from build123d import *

# Parameters (mm, degrees)
F0_R     = 1.8415
F1_DEPTH = 12.7


with BuildPart() as f1:
    # F0 (on Top) → F1 (new body, symmetric)
    with BuildSketch(Plane.XY):
        with BuildLine():
            Line((9.525, 12.7), (-9.525, 12.7))
            ThreePointArc((-9.525, 12.7), (-11.770064, 11.770064), (-12.7, 9.525))
            Line((-12.7, 9.525), (-12.7, -9.525))
            ThreePointArc((-12.7, -9.525), (-11.770064, -11.770064), (-9.525, -12.7))
            Line((-9.525, -12.7), (9.525, -12.7))
            ThreePointArc((9.525, -12.7), (11.770064, -11.770064), (12.7, -9.525))
            Line((12.7, -9.525), (12.7, 9.525))
            ThreePointArc((12.7, 9.525), (11.770064, 11.770064), (9.525, 12.7))
        make_face()
        Circle(F0_R, mode=Mode.SUBTRACT)
    extrude(amount=F1_DEPTH, both=True)


solid = f1.part
Source: CAD feature listing. Evaluate the final solid. Frame: model axes, mm. Round coordinates to 2 decimals unless told otherwise and drop trailing zeros. Loops run counter-clockwise (first coordinate to the right, second up) from the corner with the lowest first, then second, coordinate; pieces in that order, holes last.
Q1. Mould query, pull axis X, two halves, no side actions, for faces 1 (the face through (-11.79, -11.75, 0.18)), 2 (the face through (0, -12.7, 0)), 3 (the face through (0.85, -1.634, -0.178)). Classes: pulls with the +X half, pulls with the -X half, needs draft (parallel to the pull), parting line crosses it, or undercut.
Q2. Ray query, line 1 (Y direction, x = 0, z = -6.75); line 2 (Y direction, x = -9.75, z = -2.5); line 3 (X direction, y = -0.25, z = 5.75). Return the intervals inside material, ascending.
Q3. Section A-A, the plane y = 0. Return loops of the section in (x, z).
Solutions:
1. face 1: pulls with the -X half
1. face 2: needs draft
1. face 3: undercut
2. line 1: y = -12.7 to -1.84, 1.84 to 12.7
2. line 2: y = -12.69 to 12.69
2. line 3: x = -12.7 to -1.82, 1.82 to 12.7
3. outline: (-12.7, -12.7) - (-1.84, -12.7) - (-1.84, 12.7) - (-12.7, 12.7) - close; (1.84, -12.7) - (12.7, -12.7) - (12.7, 12.7) - (1.84, 12.7) - close
